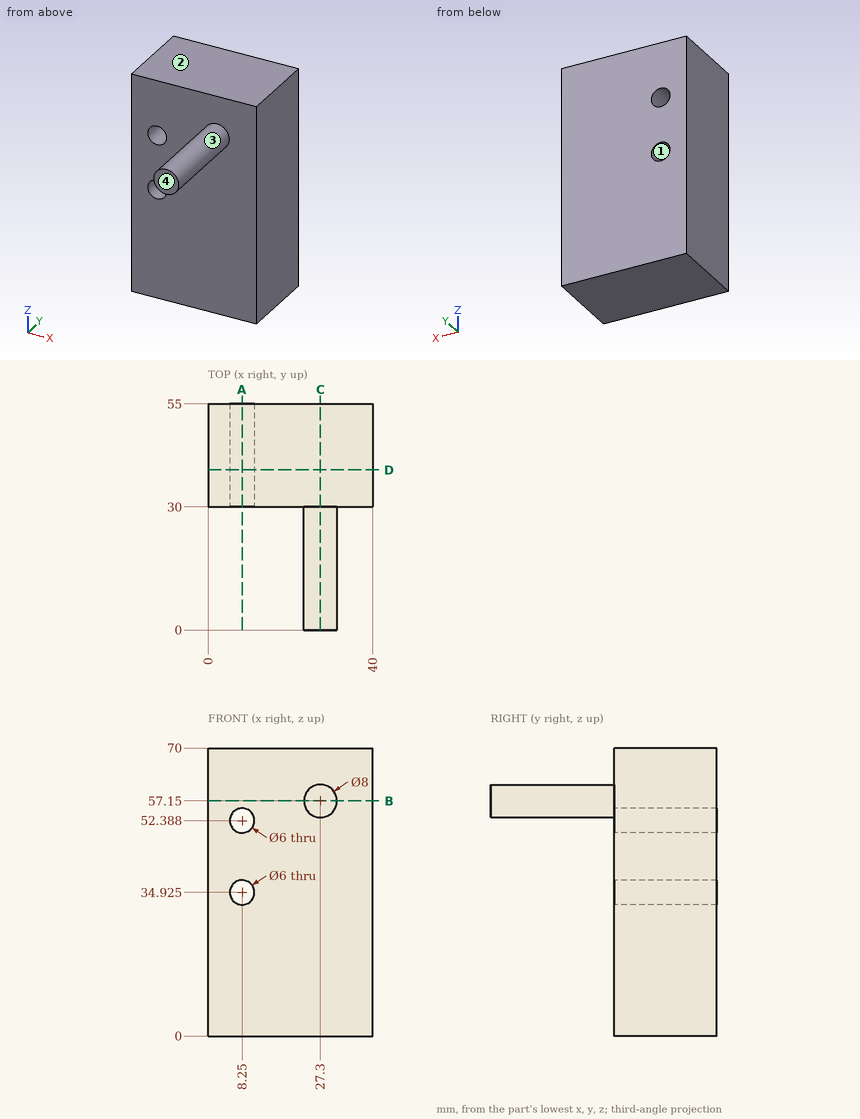
Source: three-view drawing plus pictorial views. Frame: mm from the lowest corner of the part. Coordinates: 2 decimals unless noted, no trailing zeros. Loops run counter-clockwise (first coordinate to the right, second up) from the corner with the lowest first, then second, coordinate; pieces in that order, holes last. Notation, with made-up numbers: (-7.75, 5.5) - (25.25, 5.5) arc R35 cw to (25.25, 43.5) - close; hole circle Ø2 at (-27.5, 72). An arc over 180 degrees is marked (long way). One line per question, with ' | ' between items.
1) Section C-C, the plane x = 27.3. Return loops of the section in (y, z).
Report:
outline: (0, 53.15) - (30, 53.15) - (30, 0) - (55, 0) - (55, 70) - (30, 70) - (30, 61.15) - (0, 61.15) - close
2) Section D-D, the plane y = 39. Give the number of separate pieces and of enclosed holes in the cut face, then the cut area to 3 significant figures.
Report:
separate pieces: 1 | enclosed holes: 2 | area: 2,740 mm²
3) Line query: line 1 along Z through (x, y) = (8.25, 38) (1 decimal); line 2 along Y through (x, z) = (31, 23.5); line 3 along X through (y, z) = (34, 53.5) (1 decimal). Output: solid intervals per line, ascending.
Report:
line 1: z = 0 to 31.9, 37.9 to 49.4, 55.4 to 70 | line 2: y = 30 to 55 | line 3: x = 0 to 5.5, 11 to 40
4) Section B-B, the plane z = 57.15. Return loops of the section in (x, y).
Report:
outline: (0, 30) - (23.3, 30) - (23.3, 0) - (31.3, 0) - (31.3, 30) - (40, 30) - (40, 55) - (0, 55) - close
5) Section A-A, the plane x = 8.25. Return loops of the section in (y, z) (1 decimal), then the cut area to 3 significant figures.
Report:
outline: (30, 0) - (55, 0) - (55, 31.9) - (30, 31.9) - close; (30, 37.9) - (55, 37.9) - (55, 49.4) - (30, 49.4) - close; (30, 55.4) - (55, 55.4) - (55, 70) - (30, 70) - close | area: 1,450 mm²
6) Pull-direction query (Z, two-part tool) for the marked faces 1, 2, 3 and 4; classes: released by +Z, released by -Z, zero draft, split by the parting line, or undercut.
Report:
face 1: undercut | face 2: released by +Z | face 3: split by the parting line | face 4: zero draft
7) First-contact query: P1, Ø10, axis at x = 16, z = 40.5, coming from the -Y side. Flat tip, straight axial feed; report the tip coordinate or a pass-through.
Report:
P1: stops at y = 30
